For this review, take the finished solid that the model builds, in its own axes (mm). Face numbers are marked on the shaded views. A direction names the side the tool comes from. Round coordinates to 2 decimals unless told otherwise and drop trailing zeros. Order: outer loops, then holes, each group sorted by start corner. A loop starts at its lowest first (then second) coordinate and runs counter-clockwise, first axis right, second up. Notation, with made-up numbers: (89, 44.5) - (116, 44.5) arc R26 cw to (116, 78.5) - close; hole circle Ø5 at (33.25, 23.5). An arc over 180 degrees is marked (long way). One line per item, written item: value.
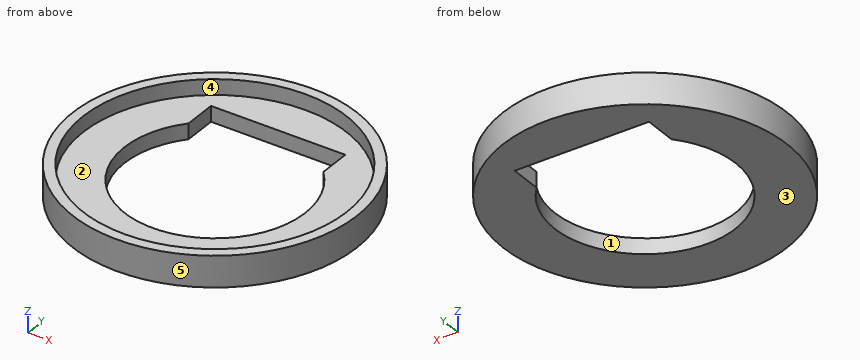
```python
from build123d import *

# Parameters (mm, degrees)
F0_R     = 27.5
F0_R_2   = 17.5
F1_DEPTH = 6
F2_R     = 25.5
F2_R_2   = 17.5
F3_DEPTH = 3
F4_W     = 26
F4_H     = 24
F5_DEPTH = 25


with BuildPart() as f1:
    # F0 (on Top) → F1 (new body)
    with BuildSketch(Plane.XY):
        Circle(F0_R)
        Circle(F0_R_2, mode=Mode.SUBTRACT)
    extrude(amount=F1_DEPTH)

    # F2 (on face) → F3 (cut)
    with BuildSketch(Plane.XY.offset(6)):
        Circle(F2_R)
        Circle(F2_R)
        Circle(F2_R_2, mode=Mode.SUBTRACT)
    extrude(amount=-F3_DEPTH, mode=Mode.SUBTRACT)

    # F4 (on face) → F5 (cut)
    with BuildSketch(Plane(origin=(0, 0, 0), x_dir=(1, 0, 0), z_dir=(0, 0, -1))):
        with Locations((-0.062166, -6)):
            Rectangle(F4_W, F4_H)
    extrude(amount=-F5_DEPTH, mode=Mode.SUBTRACT)


solid = f1.part
```
Item 1: Take a section at A-A (y = 0). Write out the cut boundary in (x, z).
Returned:
outline: (-27.5, 0) - (-17.5, 0) - (-17.5, 3) - (-25.5, 3) - (-25.5, 6) - (-27.5, 6) - close; (17.5, 0) - (27.5, 0) - (27.5, 6) - (25.5, 6) - (25.5, 3) - (17.5, 3) - close
Item 2: Take a section at C-C (z = 3.8). Write out the cut boundary in (x, y).
Returned:
outline: circle Ø55 at (0, 0); hole circle Ø51 at (0, 0)
Item 3: Wall thickness on line 1 (Y direction, x = 0, z = 1.65); line 2 (Y direction, x = 0, z = 3.9); line 3 (Z direction, x = 5, y = -24): over which ranges is each line inside the solid? List them lowest first.
Returned:
line 1: -27.5 to -17.5, 18 to 27.5
line 2: -27.5 to -25.5, 25.5 to 27.5
line 3: 0 to 3
Item 4: The part is to be moulded in two halves that separate along Y. For the marked faces 3, 4 and 5, say which applies: +Y half, -Y half, draft (parallel to the pull), parting line (faces both ways), or undercut.
Returned:
face 3: draft
face 4: undercut
face 5: parting line
Item 5: Machinability: for the marked faces 1 and 2, which of the approach directions +Z, -Z, +X, -X, +Y, -Y give a long, thin tool a straight path to every point of the face, cutting with its end or side? Answer none if there is none.
Returned:
face 1: +Z, -Z
face 2: +Z
Item 6: For P1, Ø2, axis at x = -16.5, z = 3.5, coming from the +Y side; P2, Ø1, axis at x = -2, z = 3.5, coming from the -Y side; P3, Ø1.5, axis at x = 3.5, z = 2, coming from the -Y side, all flat-tipped, find the tip position at first contact; note any pin that passes through.
Returned:
P1: y = 22.72
P2: y = -27.46
P3: y = -27.36
Item 7: Take a section at B-B (x = 0). Write out the cut boundary in (y, z), plus the area to 3 significant figures.
Returned:
outline: (-27.5, 0) - (-17.5, 0) - (-17.5, 3) - (-25.5, 3) - (-25.5, 6) - (-27.5, 6) - close; (18, 0) - (27.5, 0) - (27.5, 6) - (25.5, 6) - (25.5, 3) - (18, 3) - close
area: 70.5 mm^2
Item 8: Take a section at D-D (y = 19). Write out the cut boundary in (x, z), plus the area to 3 significant figures.
Returned:
outline: (-19.88, 0) - (19.88, 0) - (19.88, 6) - (17.01, 6) - (17.01, 3) - (-17.01, 3) - (-17.01, 6) - (-19.88, 6) - close
area: 137 mm^2
